Geometry: final body of the model. Coordinates: model frame, mm. Round coordinates to 2 decimals unless told otherwise and drop trailing zeros. Order: outer loops, then holes, each group sorted by start corner. A loop starts at its lowest first (then second) coordinate and runs counter-clockwise, first axis right, second up. Notation, with made-up numbers: M -11.5,3 L 8.5,3 A26 cw 8.5,37 Z; hole C 27,82 d2. An arc over 180 degrees is marked long. Put each result on its own line as item: value. Start each with the question number.
1) Section C-C, the plane z = 4.7. Return loops of the section in (x, y).
2) Section D-D, the plane y = 12. Return loops of the section in (x, z), then the cut area to 3 significant figures.
3) Section A-A, the plane y = 0. Return loops of the section in (x, z), then the cut area to 3 significant figures.
4) Material intervals for probe 1 along Y at (x, z) = (-86.2, 2.05); probe 2 along Y at (x, z) = (-87.5, 3.1); probe 3 along X at (y, z) = (7, 4.2), sorted ascending. Write a range as [from, to].
5) Section B-B, the plane x = -87.75. Return loops of the section in (y, z), then the cut area to 3 significant figures.
6) First-contact query: P1, Ø1, axis at x = -87.5, z = 4, coming from the +Y side; P2, Ø3, axis at y = 6, z = 1, coming from the -X side. Flat tips, straight axial feed; report the tip coordinate or a pass-through.
Autodesk Inventor part; units mm, degrees
ref_plane "YZ Plane" through (0, 0, 0) normal (1, 0, 0) x (0, 1, 0)
ref_plane "XZ Plane" through (0, 0, 0) normal (0, 1, 0) x (-1, 0, 0)
ref_plane "XY Plane" through (0, 0, 0) normal (0, 0, 1) x (1, 0, 0)
ref_plane "Arbeitsebene1" through (0, 0, 0) normal (0, 0, 1) x (1, 0, 0)
sketch "Skizze1" plane through (0, 0, 0) normal (0, 0, 1) x (1, 0, 0)
  circle A0 centre (86.2, 0) radius 2.6 construction
  circle A1 centre (-86.2, 0) radius 2.6 construction
  circle A2 centre (0, 0) radius 91.8 construction
  arc A3 (5.5, 85.9242) -> (-5.5, 85.9242) centre (0, 0) ccw construction
  line L0 (5.5, 85.9242) -> (5.5, 80.4121) construction
  arc A4 (-5.5, 80.4121) -> (5.5, 80.4121) centre (0, 0) ccw construction
  line L1 (-5.5, 80.4121) -> (-5.5, 85.9242) construction
  arc A5 (-90.4054, 15.9409) -> (-90.4054, -15.9409) centre (0, 0) ccw
  arc A6 (-79.3755, 13.996) -> (-79.3755, -13.996) centre (0, 0) ccw
  line L2 (-90.4054, 15.9409) -> (0, 0) construction
  line L3 (0, 0) -> (-90.4054, -15.9409) construction
  line L4 (-90.4054, 15.9409) -> (-79.3755, 13.996)
  line L5 (-79.3755, -13.996) -> (-90.4054, -15.9409)
  line L6 (0, 0) -> (-86.2, 0) construction
  circle A7 centre (-86.2, 0) radius 2.6
  dimension "d0" = 10
  dimension "d1" = 10
extrude "Extrusion1" add sketch "Skizze1" along normal blind 5
properties part number "Montage_Ring_Vorne_Aufdickung_Gewinde"
Result sheet:
1. outline: M -90.41,-15.94 L -79.38,-14 A80.6 cw -79.38,14 L -90.41,15.94 A91.8 ccw Z; hole C -86.2,0 d5.2
2. outline: M -91.01,0 L -79.7,0 L -79.7,5 L -91.01,5 Z
2. area: 56.6 mm2
3. outline: M -91.8,0 L -88.8,0 L -88.8,5 L -91.8,5 Z; M -83.6,0 L -80.6,0 L -80.6,5 L -83.6,5 Z
3. area: 30.0 mm2
4. probe 1: y = [-15.2, -2.6], [2.6, 15.2]
4. probe 2: y = [-15.43, -2.25], [2.25, 15.43]
4. probe 3: x = [-91.53, -80.3]
5. outline: M -15.47,0 L -2.09,0 L -2.09,5 L -15.47,5 Z; M 2.09,0 L 15.47,0 L 15.47,5 L 2.09,5 Z
5. area: 134 mm2
6. P1: stops at y = 15.52
6. P2: stops at x = -91.69
